```python
from build123d import *

# Parameters (mm, degrees)
SKETCH1_R           = 5.08
BOSS_EXTRUDE1_DEPTH = 6.35
CUT_EXTRUDE1_DEPTH  = 3.81
SKETCH3_R           = 3.1115
CUT_EXTRUDE2_DEPTH  = 2.54


with BuildPart() as part:
    # Sketch1 → Boss-Extrude1 (new body)
    with BuildSketch(Plane(origin=(0, 0, 0), x_dir=(1, 0, 0), z_dir=(0, 1, 0))):
        with Locations(Location((0, 0, 0), (0, 0, 270))):
            Circle(SKETCH1_R)
    extrude(amount=BOSS_EXTRUDE1_DEPTH)

    # Sketch2 → Cut-Extrude1 (cut)
    with BuildSketch(Plane(origin=(0, 0, 0), x_dir=(1, 0, 0), z_dir=(0, 1, 0))):
        with BuildLine():
            Line((-2.667, 1.946873134), (-2.667, -1.946873134))
            ThreePointArc((-2.667, -1.946873134), (1.023906734, -3.139238602), (3.302, 0))
            ThreePointArc((3.302, 0), (1.023906734, 3.139238602), (-2.667, 1.946873134))
        make_face()
    extrude(amount=CUT_EXTRUDE1_DEPTH, mode=Mode.SUBTRACT)

    # Sketch3 → Cut-Extrude2 (cut)
    with BuildSketch(Plane(origin=(0, 6.35, 0), x_dir=(1, 0, 0), z_dir=(0, 1, 0))):
        with Locations(Location((0, 0, 0), (0, 0, 270))):
            Circle(SKETCH3_R)
    extrude(amount=-CUT_EXTRUDE2_DEPTH, mode=Mode.SUBTRACT)


solid = part.part
```
Could you check a few things on this model? Use its own coordinates, in mm. A direction names the side the tool comes from. Coordinates: 2 decimals unless noted, no trailing zeros. Order: outer loops, then holes, each group sorted by start corner. A loop starts at its lowest first (then second) coordinate and runs counter-clockwise, first axis right, second up. Notation, with made-up numbers: M 75.25,27.25 L 107.25,27.25 A24 cw 107.25,41.25 Z; hole C 67,87 d9. An arc over 180 degrees is marked long. Use a Markdown table: item, result. Add a question column.
Q1. I want a section at A-A on x = 0. List the corners of the cut face in (y, z) for me.
Q2. We'd pull the mould along Z, two halves only. Please class faces 3 (the flat face through (-3, 0, 0)), 4 (the cylindrical face through (5.037, 3.131, -0.661)), 5 (the flat face through (-2.667, 2, 0)): pulls with the +Z half, pulls with the -Z half, needs draft (parallel to the pull), parting line crosses it, or undercut.
Q3. I want a section at D-D on x = 3.5. List the corners of the cut face in (y, z) for me, then the cut area to 3 significant figures.
Q4. I want a section at B-B on z = 1.75. List the corners of the cut face in (x, y) for me, then the cut area to 3 significant figures.
Q5. I'm going to push flat-ended pins straight in: pin 1 (2 mm diameter, centred on y = 0.5, z = -3.5, fed in from -X); pin 2 (1 mm diameter, centred on y = 3.5, z = -2.5, fed in from +X); pin 3 (2 mm diameter, centred on x = 2, z = -0.5, fed in from +Y). Where does each tip first touch, or does it pass through?
Q6. I want a section at C-C on y = 1.75. List the corners of the cut face in (x, z) for me, then the cut area to 3 significant figures.
Q7. Which directions (+Z, -Z, +X, -X, +Y, -Y) give clear straight access to the entire face, cutting with the end or side of a thin tool? Please do faces 1 (the cylindrical face through (-3.04, 5.1, -0.67)), 2 (the flat face through (-3.3, 6.35, -0.1)).
Q8. If I drill on L1, parallel to X at y = 4.95, z = 0; L2, parallel to Z at x = 0.25, y = 0.75; L3, parallel to X at y = 4.25, z = 2.5, over which ranges is the centre line in solid material (lowest first)?
Checked values:
| question | item | result |
|---|---|---|
| 1 | outline | M 0,-5.08 L 6.35,-5.08 L 6.35,-3.11 L 3.81,-3.11 L 3.81,-3.3 L 0,-3.3 Z; M 0,3.3 L 3.81,3.3 L 3.81,3.11 L 6.35,3.11 L 6.35,5.08 L 0,5.08 Z |
| 2 | face 3 | needs draft |
| 2 | face 4 | parting line crosses it |
| 2 | face 5 | undercut |
| 3 | outline | M 0,-3.68 L 6.35,-3.68 L 6.35,3.68 L 0,3.68 Z |
| 3 | area | 46.8 mm² |
| 4 | outline | M -4.77,0 L -2.67,0 L -2.67,3.81 L -2.57,3.81 L -2.57,6.35 L -4.77,6.35 Z; M 2.57,3.81 L 2.8,3.81 L 2.8,0 L 4.77,0 L 4.77,6.35 L 2.57,6.35 Z |
| 4 | area | 26.7 mm² |
| 5 | pin 1 | x = -4.42 |
| 5 | pin 2 | x = 4.67 |
| 5 | pin 3 | through |
| 6 | outline | C 0,0 d10.16; hole M -2.67,-1.95 A3.3 ccw long -2.67,1.95 Z |
| 6 | area | 48.5 mm² |
| 7 | face 1 | +Y |
| 7 | face 2 | +Z, -Z, +X, -X, +Y |
| 8 | L1 | -5.08 to -3.11, 3.11 to 5.08 |
| 8 | L2 | -5.07 to -3.29, 3.29 to 5.07 |
| 8 | L3 | -4.42 to -1.85, 1.85 to 4.42 |
